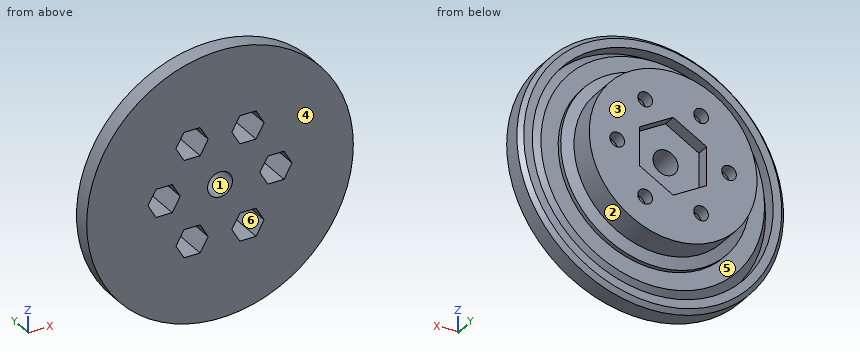
```python
from build123d import *

# Parameters (mm, degrees)
CUT_EXTRUDE_1_DEPTH = 10
HOLE_WIZARD_M31_D   = 3.4
SKETCH_10_W         = 3
SKETCH_10_H         = 3
CHAMFER_3_SIZE      = 1
CUT_EXTRUDE_2_DEPTH = 3
HOLE_WIZARD_M51_D   = 5.8


with BuildPart() as part:
    # Эскиз2 → Повернуть1 (revolve)
    with BuildSketch(Plane.XY, mode=Mode.PRIVATE) as revolve_1_sk:
        Polygon((-19.5, 2), (-22, 1), (-22, 0), (0, 0), (0, 8), (-19.5, 8), align=None)
    revolve(revolve_1_sk.sketch.rotate(Axis((0, 8, 0), (0, -1, 0)), 270), axis=Axis((0, 8, 0), (0, -1, 0)))

    # Эскиз4 → Повернуть2 (revolve)
    with BuildSketch(Plane.XY, mode=Mode.PRIVATE) as revolve_2_sk:
        Polygon((0, 0), (26, 0), (28, -3), (31, -3), (31, -5), (0, -5), (0, -3), align=None)
    revolve(revolve_2_sk.sketch.rotate(Axis((0, -3, 0), (0, -1, 0)), 180), axis=Axis((0, -3, 0), (0, -1, 0)))

    # Эскиз6 → Вырез-Вытянуть1 (cut)
    with BuildSketch(Plane.XZ.offset(5)):
        Polygon((2.74722325, -11.258330249), (4.623611625, -14.508330249), (8.376388375, -14.508330249), (10.25277675, -11.258330249), (8.376388375, -8.008330249), (4.623611625, -8.008330249), align=None)
        Polygon((-10.25277675, -11.258330249), (-8.376388375, -14.508330249), (-4.623611625, -14.508330249), (-2.74722325, -11.258330249), (-4.623611625, -8.008330249), (-8.376388375, -8.008330249), align=None)
        Polygon((-16.75277675, 0), (-14.876388375, -3.25), (-11.123611625, -3.25), (-9.24722325, 0), (-11.123611625, 3.25), (-14.876388375, 3.25), align=None)
        Polygon((-10.25277675, 11.258330249), (-8.376388375, 8.008330249), (-4.623611625, 8.008330249), (-2.74722325, 11.258330249), (-4.623611625, 14.508330249), (-8.376388375, 14.508330249), align=None)
        Polygon((2.74722325, 11.258330249), (4.623611625, 8.008330249), (8.376388375, 8.008330249), (10.25277675, 11.258330249), (8.376388375, 14.508330249), (4.623611625, 14.508330249), align=None)
        Polygon((9.24722325, 0), (11.123611625, -3.25), (14.876388375, -3.25), (16.75277675, 0), (14.876388375, 3.25), (11.123611625, 3.25), align=None)
    extrude(amount=-CUT_EXTRUDE_1_DEPTH, mode=Mode.SUBTRACT)

    # Отверстие с зазором M31 (through all)
    with Locations(Plane(origin=(0, 5, 0), x_dir=(-1, 0, 0), z_dir=(0, -1, 0))):
        with Locations((6.5, -11.258330249), (13, 0), (6.5, 11.258330249), (-6.5, 11.258330249), (-13, 0), (-6.5, -11.258330249)):
            Hole(HOLE_WIZARD_M31_D / 2)

    # Эскиз10 → Повернуть3 (revolve)
    with BuildSketch(Plane.XY, mode=Mode.PRIVATE) as revolve_3_sk:
        with Locations((-29.5, -1.5)):
            Rectangle(SKETCH_10_W, SKETCH_10_H)
    revolve(revolve_3_sk.sketch.rotate(Axis((0, -2.994452998, 0), (0, 1, 0)), 270), axis=Axis((0, -2.994452998, 0), (0, 1, 0)))

    # Фаска3
    chamfer_3_edges = [part.edges().sort_by_distance(p)[0] for p in [
        (0, 0, 31),
    ]]
    chamfer(chamfer_3_edges, length=CHAMFER_3_SIZE)

    # Эскиз11 → Вырез-Вытянуть2 (cut)
    with BuildSketch(Plane(origin=(0, 8, 0), x_dir=(1, 0, 0), z_dir=(0, 1, 0))):
        Polygon((7.794228634, -4.5), (7.794228634, 4.5), (0, 9), (-7.794228634, 4.5), (-7.794228634, -4.5), (0, -9), align=None)
    extrude(amount=-CUT_EXTRUDE_2_DEPTH, mode=Mode.SUBTRACT)

    # Отверстие с зазором M51 (through all)
    with Locations(Plane(origin=(0, -5, 0), x_dir=(-1, 0, 0), z_dir=(0, -1, 0))):
        with Locations((0, 0)):
            Hole(HOLE_WIZARD_M51_D / 2)


solid = part.part
```
Part model, mm, in its own coordinate system. Face numbers are marked on the shaded views. A direction names the side the tool comes from. Round coordinates to 2 decimals unless told otherwise and drop trailing zeros.
1. 3-axis set-ups, long thin cutter, end or side, ignore diameter. For the marked faces 4, 5 and 6: which of +Z, -Z, +X, -X, +Y, -Y reach the whole face in a straight line?
Solutions:
face 4: +Z, -Z, +X, -X, -Y
face 5: +Y
face 6: -Y
2. Drill centre lines: line 1 along X through (y, z) = (6.75, -1); line 2 along Z through (x, y) = (-6.5, 5.8); line 3 along X through (y, z) = (3.5, -3). Where is each one in solid material? Low to high.
Solutions:
line 1: x = -19.47 to -14.37, -11.63 to -7.79, 7.79 to 11.63, 14.37 to 19.47
line 2: z = -18.38 to -12.96, -9.56 to -5.25, 5.25 to 9.56, 12.96 to 18.38
line 3: x = -19.27 to -15.02, -10.98 to 10.98, 15.02 to 19.27
3. Two-plate mould, pull along X, no slides. Class the marked faces 1, 2 and 3: pulls with the +X half, pulls with the -X half, needs draft (parallel to the pull), parting line crosses it, or undercut.
Solutions:
face 1: undercut
face 2: parting line crosses it
face 3: needs draft
4. Flat gauge pins, fed straight in: pin 1 (6 mm diameter, centred on x = -14.5, y = 6, fed in from -Z); pin 2 (5 mm diameter, centred on x = -11, z = -1.5, fed in from -Y); pin 3 (1 mm diameter, centred on y = -1, z = -8, fed in from +X); pin 4 (1.9 mm diameter, centred on x = 7, y = 0.5, fed in from +Z). Where does each tip first touch, or does it go through?
Solutions:
pin 1: stops at z = -15.75
pin 2: stops at y = -5
pin 3: stops at x = 30.08
pin 4: stops at z = 29.66
5. Slice it at A-A (y = -2). Count the separate pieces of the cut face and the enclosed holes in it, and give its area (3 significant figures).
Solutions:
separate pieces: 2
enclosed holes: 8
area: 2,660 mm2
